Input: part model. Units: mm. Frame: model coordinates. Face numbers are marked on the shaded views. A direction names the side the tool comes from. Give positions to 0.01 mm unless a question says otherwise; leave off trailing zeros. Loops run counter-clockwise (first coordinate to the right, second up) from the corner with the lowest first, then second, coordinate; pieces in that order, holes last.
from build123d import *

# Parameters (mm, degrees)
F0_W     = 116.791695822
F0_H     = 79.9650549889
F1_DEPTH = 50.8
F3_DEPTH = 25.4


with BuildPart() as f1:
    # F0 (on Top) → F1 (new body)
    with BuildSketch(Plane.XY):
        with Locations((-0.9046609048, 1.5669167042)):
            Rectangle(F0_W, F0_H)
    extrude(amount=F1_DEPTH)

    # F2 (on face) → F3 (join)
    with BuildSketch(Plane.XY.offset(50.8)):
        Polygon((26.3261360564, -38.4156107903), (-25.3022870765, -38.4156107903), (1.8093218096, -83.0988883972), align=None)
        Polygon((-0.9046609047, 41.5494441986), (-59.3005088158, 40.2779845768), (-59.3005088158, 17.6176547568), (-25.3022870765, -38.4156107903), (26.3261360564, -38.4156107903), (57.4911870062, 18.3844534107), (57.4911870062, 41.5494441986), align=None)
        Polygon((71.0610874735, 43.1163628493), (-0.9046609047, 41.5494441986), (57.4911870062, 41.5494441986), (57.4911870062, 18.3844534107), align=None)
        Polygon((-59.3005088158, 40.2779845768), (-72.870409283, 39.9825255479), (-59.3005088158, 17.6176547568), align=None)
    extrude(amount=F3_DEPTH)


solid = f1.part
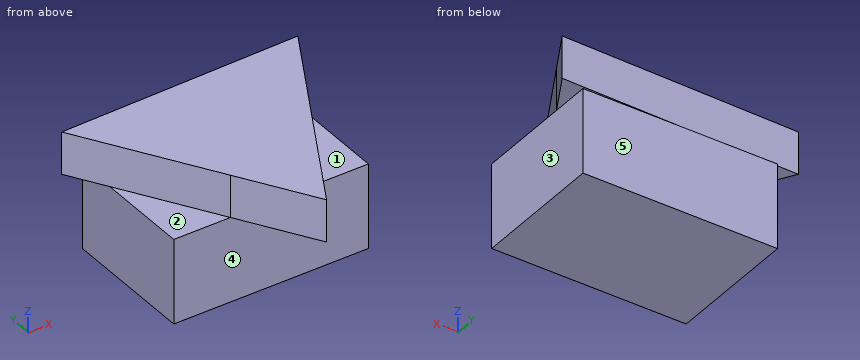
(1) Cut plane D-D (z = 33). Return the cut outline in (x, y), and give its area (3 significant figures).
Values follow:
outline: (-59.3, -38.42) - (57.49, -38.42) - (57.49, 41.55) - (-59.3, 41.55) - close
area: 9,340 mm2
(2) Ray query, probe 1 along Z at (x, y) = (-1, -46.5); probe 2 along X at (y, z) = (16, 21); probe 3 along Y at (x, z) = (-50, 26). Return the intervals inside material, ascending.
Values follow:
probe 1: z = 50.8 to 76.2
probe 2: x = -59.3 to 57.49
probe 3: y = -38.42 to 41.55
(3) Reachability of the marked faces 1, 2, 3, 4 and 5 from +Z, -Z, +X, -X, +Y, -Y: full face, straight path, thin tool, end or side. Return the list, or none.
Values follow:
face 1: +Z, +X, -Y
face 2: +Z, -X, -Y
face 3: -Z, +X, +Y, -Y
face 4: -Z, +X, -X, -Y
face 5: -Z, +X, -X, +Y
(4) Cut plane C-C (x = 35). Return the cut outline in (y, z).
Values follow:
outline: (-38.42, 0) - (41.55, 0) - (41.55, 50.8) - (42.33, 50.8) - (42.33, 76.2) - (-22.61, 76.2) - (-22.61, 50.8) - (-38.42, 50.8) - close
(5) Pin query (flat end, axial travel): pin 1 Ø10 at (x, z) = (-38.5, 21.5) entering from +Y; pin 2 Ø5 at (y, z) = (-54.5, 55.5) entering from +X; pin 3 Ø22.5 at (x, y) = (-3, -60.5) entering from -Z. Return the tip coordinate at first contact, or that it passes through.
Values follow:
pin 1: stops at y = 41.55
pin 2: stops at x = 18.87
pin 3: stops at z = 50.8
(6) Cut plane A-A (z = 70). Return the cut outline in (x, y).
Values follow:
outline: (-72.87, 39.98) - (1.81, -83.1) - (71.06, 43.12) - close
(7) Cut plane B-B (y = -24.5). Return the cut outline in (x, z).
Values follow:
outline: (-59.3, 0) - (57.49, 0) - (57.49, 50.8) - (33.96, 50.8) - (33.96, 76.2) - (-33.75, 76.2) - (-33.75, 50.8) - (-59.3, 50.8) - close
